Check sheet for the modelled part. Datum: model origin and axes. Units: mm. Face numbers are marked on the shaded views. Round coordinates to 2 decimals unless told otherwise and drop trailing zeros. Answer in a Markdown table with one row per item. Add a question column.
(1) Cross-section at A-A on z = 34. Count the separate pieces of the cut face and the enclosed holes in it, then the cut area to 3 significant figures.
(2) Thickness scan on line 1 along Y through (x, z) = (-35, 8.5); line 2 along X through (y, z) = (-7.5, 33); line 3 along X through (y, z) = (-37, 23.5). Record the ranges inside material, lowest first.
(3) Gauge pin test, flat ends, axial feed: pin 1 (1.5 mm diameter, centred on y = 76.5, z = 43.5, fed in from -X); pin 2 (1 mm diameter, centred on x = 40.5, y = -63.5, fed in from -Z); pin 3 (2.5 mm diameter, centred on y = -76.5, z = 43, fed in from +X). Record the tip position at first contact, or that the pin passes through.
(4) Mould release check, pull along X, two halves, no side actions. Record for the marked faces 1, 2 and 3: +X half, -X half, draft (parallel to the pull), parting line (faces both ways), or undercut.
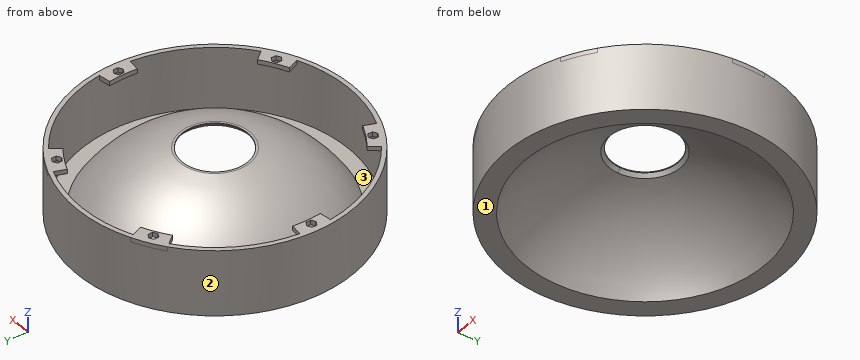
from build123d import *

# Parameters (mm, degrees)
SKETCH002_W           = 150
SKETCH002_H           = 20
POCKET_DEPTH          = 50
SKETCH001_R           = 22.5
POCKET001_DEPTH       = 45.001
PAD_DEPTH             = 3
POLARPATTERN_COUNT    = 6
POCKET002_DEPTH       = 5
POLARPATTERN001_COUNT = 6
CHAMFER_SIZE          = 2


with BuildPart() as part:
    # Sketch → Revolution (revolve)
    with BuildSketch(Plane.XZ):
        with BuildLine():
            Line((-95, 45), (-95, 0))
            Line((-95, 0), (-82, 0))
            ThreePointArc((0, 45), (-46.768045, 33.010659), (-82, 0))
            Line((0, 45), (0, 48))
            ThreePointArc((0, 48), (-46.768045, 36.010659), (-82, 3))
            Line((-82, 3), (-92, 3))
            Line((-92, 3), (-92, 45))
            Line((-92, 45), (-95, 45))
        make_face()
    revolve(axis=Axis((0, 0, 0), (0, 0, 1)))

    # Sketch002 → Pocket (cut, symmetric)
    with BuildSketch(Plane.XZ):
        with Locations((0, 55)):
            Rectangle(SKETCH002_W, SKETCH002_H)
    extrude(amount=POCKET_DEPTH, both=True, mode=Mode.SUBTRACT)

    # Sketch001 → Pocket001 (cut, through all)
    with BuildSketch(Plane.XY):
        Circle(SKETCH001_R)
    extrude(amount=POCKET001_DEPTH, mode=Mode.SUBTRACT)

    # Sketch003 → Pad (join)
    with BuildSketch(Plane.XY.offset(45)):
        with BuildLine():
            ThreePointArc((-94.347763, 11.113041), (-95, 0), (-94.347763, -11.113041))
            Line((-83.480776, -9.563365), (-94.347763, -11.113041))
            ThreePointArc((-83.480776, 9.563365), (-84.020478, 0), (-83.480776, -9.563365))
            Line((-83.480776, 9.563365), (-94.347763, 11.113041))
        make_face()
    pad = extrude(amount=-PAD_DEPTH)

    # PolarPattern: Pad ×6 about axis
    polarpattern_axis = Axis((0, 0, 0), (0, 0, 1))
    for i in range(1, POLARPATTERN_COUNT):
        add(pad.rotate(polarpattern_axis, i * 360 / POLARPATTERN_COUNT))

    # Sketch004 → Pocket002 (cut)
    with BuildSketch(Plane.XY.offset(45)):
        Polygon((-85.185417, 1.625), (-88, 3.25), (-90.814583, 1.625), (-90.814583, -1.625), (-88, -3.25), (-85.185417, -1.625), align=None)
    pocket002 = extrude(amount=-POCKET002_DEPTH, mode=Mode.SUBTRACT)

    # PolarPattern001: Pocket002 ×6 about axis
    polarpattern001_axis = Axis((0, 0, 0), (0, 0, 1))
    for i in range(1, POLARPATTERN001_COUNT):
        add(pocket002.rotate(polarpattern001_axis, i * 360 / POLARPATTERN001_COUNT), mode=Mode.SUBTRACT)

    # Chamfer
    chamfer_edges = [part.edges().sort_by_distance(p)[0] for p in [
        (0, 22.5, 42.360291),
        (0, -22.5, 42.360291),
    ]]
    chamfer(chamfer_edges, length=CHAMFER_SIZE)


solid = part.part
Answers:
| question | item | result |
|---|---|---|
| 1 | separate pieces | 2 |
| 1 | enclosed holes | 2 |
| 1 | area | 3,360 mm^2 |
| 2 | line 1 | y = -88.32 to -85.08, -69.96 to -67.37, 67.37 to 69.96, 85.08 to 88.32 |
| 2 | line 2 | x = -94.7 to -91.69, -51.33 to -46.18, 46.18 to 51.33, 91.69 to 94.7 |
| 2 | line 3 | x = -87.5 to -84.23, -52.86 to -48.46, 48.46 to 52.86, 84.23 to 87.5 |
| 3 | pin 1 | stops at x = -57.33 |
| 3 | pin 2 | stops at z = 8.63 |
| 3 | pin 3 | stops at x = 57.99 |
| 4 | face 1 | draft |
| 4 | face 2 | parting line |
| 4 | face 3 | undercut |
